Check sheet for the modelled part. Datum: model origin and axes. Units: mm. A direction names the side the tool comes from. Coordinates: 2 decimals unless noted, no trailing zeros. Write each loop counter-clockwise with the first axis right and the second up, starting at its lowest first coordinate (ties: lowest second). Pieces come first, ordered by that corner, then holes. Notation, with made-up numbers: (-9, 22) -> (-3, 22) arc R14 cw to (-3, 30) -> close; hole circle Ø6 at (69, 56.25). An arc over 180 degrees is marked (long way). One line per item, written item: value. Start each with the question number.
1) Gauge pin test, flat ends, axial feed: P1, Ø10, axis at x = 79.5, y = 15, coming from the -Z side; P2, Ø10.5, axis at x = 47, y = 13.5, coming from the +Z side; P3, Ø10, axis at x = 106.5, y = -19.5, coming from the -Z side. Record the tip position at first contact, or that the pin passes through.
2) Set-up check for faces 4 (the cylindrical face through (61.17, 20.15, -19.94)), 5 (the cylindrical face through (61.17, -20.15, -19.94)), 6 (the cylindrical face through (27.69, 14.22, -138.82)), 7 (the cylindrical face through (92.96, -14.22, -38.98)), 8 (the cylindrical face through (59.48, -9.66, -165.2)): record each of +Z, -Z, +X, -X, +Y, -Y from which the full face is reachable in a straight line by a thin tool's end or side.
3) Sectioned sample at C-C on y = 0. Enter the section's corners in (x, z) (3 decimals).
4) Sectioned sample at A-A on z = -177.8. Enter the section's corners in (x, y) (3 decimals).
5) Draft check along X on faces 1 (the cylindrical face through (59.48, -15.497, 3.441)), 2 (the cylindrical face through (93.077, 14.221, -138.705)), 3 (the flat face through (120.65, 0, -87)). Enter one of: +X half, -X half, draft (parallel to the pull), parting line (faces both ways), or undercut.
6) Sectioned sample at B-B on x = 48. Enter the section's corners in (y, z) (3 decimals), plus the area to 3 significant figures.
7) Sectioned sample at D-D on y = -12.5. Enter the section's corners in (x, z), plus the area to 3 significant figures.
8) Scan lines: line 1 along Z through (x, y) = (94.5, 0) (3 decimals); line 2 along Y through (x, z) = (53.5, -177.8) (3 decimals); line 3 along Z through (x, y) = (113.5, 10). Record each from-to range of solid material in increasing order. Write a range as [from, to].
```python
from build123d import *

# Parameters (mm, degrees)
SKETCH1_R               = 15.875
BOSS_EXTRUDE1_DEPTH     = 127
FILLET1_R               = 50.8
SKETCH2_W               = 25.4
SKETCH2_H               = 241.689615924
CUT_EXTRUDE1_DEPTH      = 7.35
CUT_EXTRUDE1_DEPTH_BACK = 45.45
SKETCH3_W               = 69.85
SKETCH3_H               = 104.192939654
CUT_EXTRUDE2_DEPTH      = 9.525
FILLET2_R               = 7.62
FILLET2_OF_MIRROR1_R    = 7.62


with BuildPart() as part:
    # Sketch1 → Boss-Extrude1 (new body)
    with BuildSketch(Plane(origin=(0, 0, 0), x_dir=(0, 0, -1), z_dir=(1, 0, 0))):
        with BuildLine():
            ThreePointArc((16.800520825, 19.05), (-25.4, 0), (16.800520825, -19.05))
            Line((16.800520825, -19.05), (160.999479175, -19.05))
            ThreePointArc((160.999479175, -19.05), (203.2, 0), (160.999479175, 19.05))
            Line((160.999479175, 19.05), (16.800520825, 19.05))
        make_face()
        Circle(SKETCH1_R, mode=Mode.SUBTRACT)
        with Locations((177.8, 0)):
            Circle(SKETCH1_R, mode=Mode.SUBTRACT)
    extrude(amount=BOSS_EXTRUDE1_DEPTH)

    # Fillet1
    fillet1_edges = [part.edges().sort_by_distance(p)[0] for p in [
        (63.5, -19.05, -16.800520825),
        (63.5, 19.05, -16.800520825),
        (63.5, 19.05, -160.999479175),
        (63.5, -19.05, -160.999479175),
    ]]
    fillet(fillet1_edges, radius=FILLET1_R)

    # Sketch2 → Cut-Extrude1 (cut, two sides)
    with BuildSketch(Plane(origin=(0, 19.05, 0), x_dir=(1, 0, 0), z_dir=(0, 1, 0))) as cut_extrude1_sk:
        with Locations((133.35, 89.453065483)):
            Rectangle(SKETCH2_W, SKETCH2_H)
    extrude(amount=CUT_EXTRUDE1_DEPTH, mode=Mode.SUBTRACT)
    extrude(cut_extrude1_sk.sketch, amount=-CUT_EXTRUDE1_DEPTH_BACK, mode=Mode.SUBTRACT)

    # Sketch3 → Cut-Extrude2 (cut)
    with BuildSketch(Plane(origin=(0, 19.05, 0), x_dir=(1, 0, 0), z_dir=(0, 1, 0))):
        with Locations((60.325, 88.9)):
            Rectangle(SKETCH3_W, SKETCH3_H)
    cut_extrude2 = extrude(amount=-CUT_EXTRUDE2_DEPTH, mode=Mode.SUBTRACT)

    # Fillet2
    fillet2_edges = [part.edges().sort_by_distance(p)[0] for p in [
        (25.4, 14.2875, -36.803530173),
        (25.4, 14.2875, -140.996469827),
        (95.25, 14.2875, -140.996469827),
        (95.25, 14.2875, -36.803530173),
    ]]
    fillet(fillet2_edges, radius=FILLET2_R)

    # Mirror1: Cut-Extrude2 across plane
    add(cut_extrude2.mirror(Plane.ZX), mode=Mode.SUBTRACT)

    # Fillet2 of Mirror1
    fillet2_of_mirror1_edges = [part.edges().sort_by_distance(p)[0] for p in [
        (25.4, -14.2875, -36.803530173),
        (25.4, -14.2875, -140.996469827),
        (95.25, -14.2875, -140.996469827),
        (95.25, -14.2875, -36.803530173),
    ]]
    fillet(fillet2_of_mirror1_edges, radius=FILLET2_OF_MIRROR1_R)


solid = part.part
```
Answers:
1. P1: stops at z = -201.15
1. P2: stops at z = 24.02
1. P3: stops at z = -198.65
2. face 4: +X, -X, +Y
2. face 5: +X, -X, -Y
2. face 6: +Y
2. face 7: -Y
2. face 8: +X, -X
3. outline: (0, -203.2) -> (120.65, -203.2) -> (120.65, -193.675) -> (0, -193.675) -> close; (0, -161.925) -> (120.65, -161.925) -> (120.65, -15.875) -> (0, -15.875) -> close; (0, 15.875) -> (120.65, 15.875) -> (120.65, 25.4) -> (0, 25.4) -> close
4. outline: (0, -25.4) -> (120.65, -25.4) -> (120.65, -15.875) -> (0, -15.875) -> close; (0, 15.875) -> (120.65, 15.875) -> (120.65, 25.4) -> (0, 25.4) -> close
5. face 1: draft
5. face 2: undercut
5. face 3: +X half
6. outline: (-23.283, -167.649) arc R25.4 ccw (long way) to (23.283, -167.649) arc R50.8 cw to (19.05, -147.346) -> (19.05, -140.996) -> (9.525, -140.996) -> (9.525, -36.804) -> (19.05, -36.804) -> (19.05, -30.454) arc R50.8 cw to (23.283, -10.151) arc R25.4 ccw (long way) to (-23.283, -10.151) arc R50.8 cw to (-19.05, -30.454) -> (-19.05, -36.804) -> (-9.525, -36.804) -> (-9.525, -140.996) -> (-19.05, -140.996) -> (-19.05, -147.346) arc R50.8 cw to start; hole circle Ø31.75 at (0, -177.8); hole circle Ø31.75 at (0, 0)
6. area: 5,570 mm2
7. outline: (0, -199.91) -> (120.65, -199.91) -> (120.65, -187.59) -> (0, -187.59) -> close; (0, -168.01) -> (120.65, -168.01) -> (120.65, -9.79) -> (0, -9.79) -> close; (0, 9.79) -> (120.65, 9.79) -> (120.65, 22.11) -> (0, 22.11) -> close; hole (25.4, -133.38) arc R7.62 ccw to (33.02, -141) -> (87.63, -141) arc R7.62 ccw to (95.25, -133.38) -> (95.25, -44.42) arc R7.62 ccw to (87.63, -36.8) -> (33.02, -36.8) arc R7.62 ccw to (25.4, -44.42) -> close
7. area: 14,800 mm2
8. line 1: z = [-203.2, -193.675], [-161.925, -15.875], [15.875, 25.4]
8. line 2: y = [-25.4, -15.875], [15.875, 25.4]
8. line 3: z = [-201.15, -190.13], [-165.47, -12.33], [12.33, 23.35]
